from build123d import *

# Parameters (mm, degrees)
BOSS_EXTRUDE2_DEPTH = 250
BOSS_EXTRUDE3_DEPTH = 25
CUT_EXTRUDE1_DEPTH  = 20
BOSS_EXTRUDE4_DEPTH = 25
CUT_EXTRUDE2_DEPTH  = 20
SKETCH6_R           = 10
SKETCH6_R_2         = 1.7
BOSS_EXTRUDE5_DEPTH = 5


with BuildPart() as part:
    # Sketch1 → Boss-Extrude2 (new body)
    with BuildSketch(Plane(origin=(0, 0, 0), x_dir=(0, 0, -1), z_dir=(1, 0, 0))):
        Polygon((-30.524745156, -8.565955709), (67.5, 35.000597694), (165.524745156, -8.565955709), (165.524745156, -13.566553403), (135, 0), (67.5, 30), (0, 0), (-30.524745156, -13.566553403), align=None)
    extrude(amount=-BOSS_EXTRUDE2_DEPTH)

    # Sketch2 → Boss-Extrude3 (add)
    with BuildSketch(Plane(origin=(0, 0, 0), x_dir=(0, 0, -1), z_dir=(1, 0, 0))):
        Polygon((0, 0), (135, 0), (67.5, 30), align=None)
    extrude(amount=-BOSS_EXTRUDE3_DEPTH)

    # Sketch3 → Cut-Extrude1 (cut)
    with BuildSketch(Plane(origin=(0, 0, 0), x_dir=(0, 0, -1), z_dir=(1, 0, 0))):
        Polygon((0, 0), (135, 0), (67.5, 30), align=None)
    extrude(amount=-CUT_EXTRUDE1_DEPTH, mode=Mode.SUBTRACT)

    # Sketch4 → Boss-Extrude4 (add)
    with BuildSketch(Plane.ZY.offset(250)):
        Polygon((0, 0), (-135, 0), (-67.5, 30), align=None)
    extrude(amount=-BOSS_EXTRUDE4_DEPTH)

    # Sketch5 → Cut-Extrude2 (cut)
    with BuildSketch(Plane.ZY.offset(250)):
        Polygon((-135, 0), (0, 0), (-67.5, 30), align=None)
    extrude(amount=-CUT_EXTRUDE2_DEPTH, mode=Mode.SUBTRACT)

    # Sketch6 → Boss-Extrude5 (add)
    # profile 1 of 2: a face of its own
    with BuildSketch(Plane(origin=(0, 0, 0), x_dir=(-1, 0, 0), z_dir=(0, -1, 0))):
        with Locations((230, 67.5)):
            Circle(SKETCH6_R)
        with Locations(Location((235, 67.5, 0), (0, 0, 90))):
            Circle(SKETCH6_R_2, mode=Mode.SUBTRACT)
    # profile 2 of 2: a face of its own
    with BuildSketch(Plane(origin=(0, 0, 0), x_dir=(-1, 0, 0), z_dir=(0, -1, 0))):
        with Locations((20, 67.5)):
            Circle(SKETCH6_R)
        with Locations(Location((15, 67.5, 0), (0, 0, 90))):
            Circle(SKETCH6_R_2, mode=Mode.SUBTRACT)
    extrude(amount=-BOSS_EXTRUDE5_DEPTH)


solid = part.part
Verification items for the finished model (mm, model axes). A direction names the side the tool comes from. Give positions to 0.01 mm unless a question says otherwise; leave off trailing zeros. Loops run counter-clockwise (first coordinate to the right, second up) from the corner with the lowest first, then second, coordinate; pieces in that order, holes last. Notation, with made-up numbers: (-20, -21.75) - (14, -21.75) arc R32 ccw to (14, 13.25) - close; hole circle Ø10 at (-19.75, 81). An arc over 180 degrees is marked (long way). Write item = value, one per line. Start each with the question number.
Q1. Cross-section at C-C, the plane z = -93. Enter the section's corners in (x, y), and give its area (3 significant figures).
Q2. Tool access check on faces 5 (the face through (-17, 5, -68)), 6 (the face through (-10, 2.5, -67.7)), 7 (the face through (-225, 12, -67)), 8 (the face through (-230, 12, -68)), 9 (the face through (-240, 2.5, -67.3)). Record the directions out of +Z, -Z, +X, -X, +Y, -Y that give a thin tool (end or side, any length) a straight path to the whole face; none if there is none.
Q3. Cross-section at A-A, the plane x = -89. Enter the section's corners in (y, z), and give its area (3 significant figures).
Q4. Depth check by flat-ended pin: P1, Ø4.5, axis at x = -15, z = -67.5, coming from the -Y side; P2, Ø1.5, axis at x = -144.5, z = -116, coming from the +Y side; P3, Ø4, axis at x = -169.5, z = -110.5, coming from the +Y side. Enter the tip coordinate at first touch or a pass-through.
Q5. Cross-section at D-D, the plane z = -138.5. Enter the section's corners in (x, y).
Q6. Thickness scan on line 1 (X direction, y = 2.7, z = -67.5); line 2 (Z direction, x = -235, y = 1); line 3 (Z direction, x = -235, y = 1.4). Record the ranges inside material, lowest first.
Q7. Mould release check, pull along X, two halves, no side actions. Record for faces 1 (the face through (-30, 2.5, -67.4)), 2 (the face through (-220, 2.5, -67.6)), 3 (the face through (-20, 12, -67)), 4 (the face through (-228, 0, -68)): released by +X, released by -X, zero draft, split by the parting line, or undercut.
Q8. Cross-section at B-B, the plane y = 24.5. Enter the section's corners in (x, z) (3 decimals), and give its area (3 significant figures).
Answer key:
q1.outline = (-250, 18.67) - (-230, 18.67) - (-230, 0) - (-225, 0) - (-225, 18.67) - (-25, 18.67) - (-25, 0) - (-20, 0) - (-20, 18.67) - (0, 18.67) - (0, 23.67) - (-250, 23.67) - close
q1.area = 1,440 mm^2
q2.face_5 = +X
q2.face_6 = +X, -Y
q2.face_7 = none
q2.face_8 = -X
q2.face_9 = -X, -Y
q3.outline = (-13.57, -165.52) - (-8.57, -165.52) - (35, -67.5) - (-8.57, 30.52) - (-13.57, 30.52) - (30, -67.5) - close
q3.area = 980 mm^2
q4.P1 = 0
q4.P2 = 13.78
q4.P3 = 16.78
q5.outline = (-250, -1.56) - (0, -1.56) - (0, 3.45) - (-250, 3.45) - close
q6.line_1 = -240 to -236.7, -233.3 to -220, -30 to -16.7, -13.3 to -10
q6.line_2 = -144 to -132.75, -76.16 to -69.2, -65.8 to -58.84, -2.25 to 9
q6.line_3 = -143.1 to -131.85, -76.16 to -69.2, -65.8 to -58.84, -3.15 to 8.1
q7.face_1 = undercut
q7.face_2 = undercut
q7.face_3 = released by +X
q7.face_4 = zero draft
q8.outline = (-250, -91.126) - (0, -91.126) - (0, -79.875) - (-20, -79.875) - (-20, -55.125) - (0, -55.125) - (0, -43.874) - (-250, -43.874) - (-250, -55.125) - (-230, -55.125) - (-230, -79.875) - (-250, -79.875) - close; hole (-225, -79.875) - (-25, -79.875) - (-25, -55.125) - (-225, -55.125) - close
q8.area = 5,870 mm^2
